from build123d import *

# Parameters (mm, degrees)
F0_W     = 55.245
F0_H     = 8.255
F0_W_2   = 52.07
F0_H_2   = 5.08
F1_DEPTH = 52.3875
F2_DEPTH = 50.8


with BuildPart() as f1:
    # F0 (on Top) → F1 (new body)
    with BuildSketch(Plane.XY):
        Rectangle(F0_W, F0_H)
        Rectangle(F0_W_2, F0_H_2, mode=Mode.SUBTRACT)
        Rectangle(F0_W_2, F0_H_2)
    extrude(amount=-F1_DEPTH)

    # F0 (on Top) → F2 (cut)
    with BuildSketch(Plane.XY):
        Rectangle(F0_W_2, F0_H_2)
    extrude(amount=-F2_DEPTH, mode=Mode.SUBTRACT)


solid = f1.part
Verification items for the finished model (mm, model axes). A direction names the side the tool comes from. Coordinates: 2 decimals unless noted, no trailing zeros. Loops run counter-clockwise (first coordinate to the right, second up) from the corner with the lowest first, then second, coordinate; pieces in that order, holes last. Notation, with made-up numbers: M 25,6 L 65,6 A19 cw 65,11 Z; hole C 12,80.5 d5. An arc over 180 degrees is marked long. One line per item, written item: value.
1. Section check B-B on x = 24.5. Record the cut outline in (y, z), plus the area to 3 significant figures.
Answers follow:
outline: M -4.13,-52.39 L 4.13,-52.39 L 4.13,0 L 2.54,0 L 2.54,-50.8 L -2.54,-50.8 L -2.54,0 L -4.13,0 Z
area: 174 mm^2
2. Material ranges on line 1 along Y through (x, z) = (-18, -45.5); line 2 along X through (y, z) = (-0.5, -33) (1 decimal); line 3 along Z through (x, y) = (-17.5, 2.5), recorded low to high. Write a range as from..to.
Answers follow:
line 1: -4.13..-2.54, 2.54..4.13
line 2: -27.6..-26, 26..27.6
line 3: -52.39..-50.8
3. Mould release check, pull along Y, two halves, no side actions. Record for faces 1 (the flat face through (0, 4.128, -26)), 2 (the flat face through (-26.035, 0, -25)), 3 (the flat face through (27.622, 0, -26)): pulls with the +Y half, pulls with the -Y half, needs draft (parallel to the pull), parting line crosses it, or undercut.
Answers follow:
face 1: pulls with the +Y half
face 2: undercut
face 3: needs draft
4. Gauge pin test, flat end, axial feed: P1, Ø3, axis at x = -20, y = -0.5, coming from the +Z side. Record the tip position at first contact, or that the pin passes through.
Answers follow:
P1: z = -50.8
5. Section check A-A on z = -48. Record the cut outline in (x, y) (1 decimal), plus the area to 3 significant figures.
Answers follow:
outline: M -27.6,-4.1 L 27.6,-4.1 L 27.6,4.1 L -27.6,4.1 Z; hole M -26,-2.5 L 26,-2.5 L 26,2.5 L -26,2.5 Z
area: 192 mm^2
6. Section check C-C on y = 1.25. Record the cut outline in (x, z) (1 decimal).
Answers follow:
outline: M -27.6,-52.4 L 27.6,-52.4 L 27.6,0 L 26,0 L 26,-50.8 L -26,-50.8 L -26,0 L -27.6,0 Z
7. Set-up check for faces 4 (the flat face through (0, 0, -50.8)), 5 (the flat face through (0, 0, -52.388)): record each of +Z, -Z, +X, -X, +Y, -Y from which the full face is reachable in a straight line by a thin tool's end or side.
Answers follow:
face 4: +Z
face 5: -Z, +X, -X, +Y, -Y
